Build history of the part. All positions in model axes, mm. A direction names the side the tool comes from. Round coordinates to 2 decimals unless told otherwise and drop trailing zeros. Write each loop counter-clockwise with the first axis right and the second up, starting at its lowest first coordinate (ties: lowest second). Pieces come first, ordered by that corner, then holes. Notation, with made-up numbers: M 53,24.5 L 92,24.5 A24 ccw 92,52.5 Z; hole C 28,-32 d6. An arc over 180 degrees is marked long. Use a Markdown table: item, result.
from build123d import *


with BuildPart() as part:
    # Esquisse1 → Révolution1 (revolve)
    with BuildSketch(Plane.XY, mode=Mode.PRIVATE) as r_volution1_sk:
        Polygon((0, 9.5), (0, 6.25), (-2, 6.25), (-2, 2.1), (-11, 2.1), (-11, 5), (-14, 5), (-14, 7.25), (-11.5, 7.25), (-11.5, 7), (-11, 7), (-11, 7.25), (-8.5, 7.25), (-4, 7.5), (-2.5, 9), align=None)
    revolve(r_volution1_sk.sketch.rotate(Axis((-14.253108504, 0, 0), (1, 0, 0)), 90), axis=Axis((-14.253108504, 0, 0), (1, 0, 0)))  # turned: the seam where the file's is


solid = part.part
Q1. Which spindle directions (+Z, -Z, +X, -X, +Y, -Y) get a long thin tool onto all of the face, cutting with end or side? Do faces 1 (the cylindrical face through (-12.73, 6.43, 3.35)), 2 (the cylindrical face through (-11.25, 6.21, 3.23)), 3 (the flat face through (-2, 3, 0)), 4 (the flat face through (0, 6.2, 2)), 5 (the cylindrical face through (-6.563, -0.631, 2.003)). Say none if no direction does.
Response values:
| item | result |
|---|---|
| face 1 | -X |
| face 2 | none |
| face 3 | +X |
| face 4 | +Z, -Z, +X, +Y, -Y |
| face 5 | +X, -X |
Q2. Two-plate mould, pull along Z, no slides. Class faces 6 (the flat face through (-11, 1, -2.2)), 7 (the conical face through (-2.344, -2.713, 8.614)), 8 (the flat face through (-14, 5, 2)): +Z half, -Z half, draft (parallel to the pull), parting line (faces both ways), or undercut.
Response values:
| item | result |
|---|---|
| face 6 | undercut |
| face 7 | parting line |
| face 8 | draft |
Q3. Cut at D-D on x = -1.5. Give the cut face in (y, z).
Response values:
| item | result |
|---|---|
| outline | C 0,0 d18.4; hole C 0,0 d12.5 |
Q4. Cut at C-C on x = -13. Give the cut face in (y, z), and give its area (3 significant figures).
Response values:
| item | result |
|---|---|
| outline | C 0,0 d14.5; hole C 0,0 d10 |
| area | 86.6 mm2 |
Q5. Drop flat-ended pins along their axis: P1, Ø2, axis at x = -12, y = -4, coming from the +Z side; P2, Ø8, axis at x = -4, z = 7, coming from the -Y side; P3, Ø2, axis at y = -0.5, z = 2, coming from the -X side. Give the stop position or say it passes through.
Response values:
| item | result |
|---|---|
| P1 | stops at z = 6.6 |
| P2 | stops at y = -8.39 |
| P3 | stops at x = -11 |
Q6. Drill centre lines: L1, parallel to X at y = 1, z = 2.25; L2, parallel to Y at x = -11.8, z = 0; L3, parallel to Y at x = -1, z = 2. Where is each one in solid material? Low to high.
Response values:
| item | result |
|---|---|
| L1 | x = -11 to -2 |
| L2 | y = -7.25 to -5, 5 to 7.25 |
| L3 | y = -9.08 to -5.92, 5.92 to 9.08 |
